Work out the finished part from the listing and answer in its coordinate system (mm). Face numbers are marked on the shaded views. A direction names the side the tool comes from. Give positions to 0.01 mm unless a question says otherwise; leave off trailing zeros. Order: outer loops, then holes, each group sorted by start corner. A loop starts at its lowest first (then second) coordinate and runs counter-clockwise, first axis right, second up. Notation, with made-up numbers: M -18.5,14 L -14.5,14 A18 cw -14.5,40 Z; hole C 44.5,-11.75 d3. An arc over 180 degrees is marked long. One line per item, written item: value.
from build123d import *

# Parameters (mm, degrees)
SKETCH1_W             = 76.2
SKETCH1_H             = 203.2
BOSS_EXTRUDE1_DEPTH   = 6.35
BOSS_EXTRUDE1_2_DEPTH = 6.35
SKETCH2_W             = 38.1
SKETCH2_H             = 76.2
BOSS_EXTRUDE2_DEPTH   = 889
SKETCH3_W             = 177.8
SKETCH3_H             = 38.1
BOSS_EXTRUDE3_DEPTH   = 76.2
SKETCH4_R             = 4.2
CUT_EXTRUDE1_DEPTH    = 180
SKETCH5_R             = 2.6
CUT_EXTRUDE2_DEPTH    = 10
SKETCH6_W             = 25
SKETCH6_H             = 18
BOSS_EXTRUDE4_DEPTH   = 10
SKETCH7_W             = 177.8
SKETCH7_H             = 19
BOSS_EXTRUDE5_DEPTH   = 2.54


with BuildPart() as part:
    # Sketch1 → Boss-Extrude1 (new body)
    with BuildSketch(Plane(origin=(0, 0, 0), x_dir=(1, 0, 0), z_dir=(0, 1, 0))):
        with Locations((127, -101.6)):
            Rectangle(SKETCH1_W, SKETCH1_H)
    extrude(amount=BOSS_EXTRUDE1_DEPTH)



with BuildPart() as body_2:
    # Sketch1 → Boss-Extrude1 2 (new body)
    with BuildSketch(Plane(origin=(0, 0, 0), x_dir=(1, 0, 0), z_dir=(0, 1, 0))):
        with Locations((-127, -101.6)):
            Rectangle(SKETCH1_W, SKETCH1_H)
    extrude(amount=BOSS_EXTRUDE1_2_DEPTH)


with BuildPart() as part_1:
    add(part.part)

    add(body_2.part)  # Boss-Extrude2 merges body 2
    # Sketch2 → Boss-Extrude2 (add)
    with BuildSketch(Plane(origin=(0, 6.35, 0), x_dir=(1, 0, 0), z_dir=(0, 1, 0))):
        with Locations((-107.95, -101.6)):
            Rectangle(SKETCH2_W, SKETCH2_H)
        with Locations((107.95, -101.6)):
            Rectangle(SKETCH2_W, SKETCH2_H)
    extrude(amount=BOSS_EXTRUDE2_DEPTH)

    # Sketch3 → Boss-Extrude3 (add)
    with BuildSketch(Plane.XY.offset(139.7)):
        with Locations((0, 876.3)):
            Rectangle(SKETCH3_W, SKETCH3_H)
        with Locations((0, 711.2)):
            Rectangle(SKETCH3_W, SKETCH3_H)
    extrude(amount=-BOSS_EXTRUDE3_DEPTH)

    # Sketch4 → Cut-Extrude1 (cut)
    with BuildSketch(Plane(origin=(0, 895.35, 0), x_dir=(1, 0, 0), z_dir=(0, 1, 0))):
        with Locations(Location((0, -119.7, 0), (0, 0, 270))):
            Circle(SKETCH4_R)
    extrude(amount=-CUT_EXTRUDE1_DEPTH, mode=Mode.SUBTRACT)

    # Sketch5 → Cut-Extrude2 (cut)
    with BuildSketch(Plane.XZ.offset(-857.25)):
        with Locations(Location((-12, 119.7, 0), (0, 0, 270))):
            Circle(SKETCH5_R)
        with Locations(Location((12, 119.7, 0), (0, 0, 90))):
            Circle(SKETCH5_R)
    extrude(amount=-CUT_EXTRUDE2_DEPTH, mode=Mode.SUBTRACT)

    # Sketch6 → Boss-Extrude4 (add)
    with BuildSketch(Plane(origin=(0, 730.25, 0), x_dir=(1, 0, 0), z_dir=(0, 1, 0))):
        with Locations((52.5, -130.7)):
            Rectangle(SKETCH6_W, SKETCH6_H)
        with Locations((-52.5, -130.7)):
            Rectangle(SKETCH6_W, SKETCH6_H)
    extrude(amount=BOSS_EXTRUDE4_DEPTH)

    # Sketch7 → Boss-Extrude5 (add)
    with BuildSketch(Plane.XY.offset(139.7)):
        with Locations((0, 819.25)):
            Rectangle(SKETCH7_W, SKETCH7_H)
    extrude(amount=-BOSS_EXTRUDE5_DEPTH)


solid = part_1.part
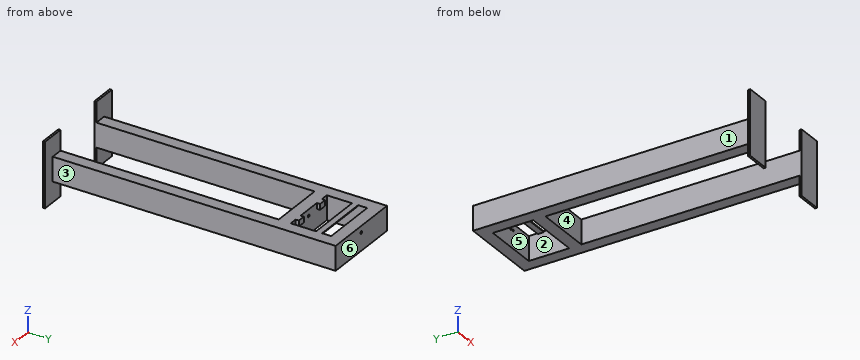
(1) Which of the six approach directions +Z, -Z, +X, -X, +Y, -Y give full straight-line access (tool end or side, diameter ignored) to the marked faces 4, 5 and 6?
Findings:
face 4: +Z, -Z, -Y
face 5: +Z, -Z
face 6: +Z, -Z, +X, -X, +Y
(2) Find the intervals of material crossed by probe 1 along X at (y, z) = (787, 65.5); probe 2 along X at (y, z) = (874, 119); probe 3 along X at (y, z) = (865, 119), in increasing order. Write a range as from..to.
Findings:
probe 1: x = -127..-88.9, 88.9..127
probe 2: x = -127..-4.14, 4.14..127
probe 3: x = -127..-14.5, -9.5..-4.14, 4.14..9.5, 14.5..127
(3) Section B-B, the plane z = 90 is taken. Give the vertices of the cut face in (x, y), then the cut area to 3 significant figures.
Findings:
outline: M -165.1,0 L -88.9,0 L -88.9,692.15 L 88.9,692.15 L 88.9,0 L 165.1,0 L 165.1,6.35 L 127,6.35 L 127,895.35 L -127,895.35 L -127,6.35 L -165.1,6.35 Z; hole M -88.9,730.25 L 88.9,730.25 L 88.9,857.25 L -88.9,857.25 Z
area: 82,300 mm^2
(4) Section C-C, the plane z = 173.5 is taken. Give the vertices of the cut face in (x, y), then the cut area to 3 significant figures.
Findings:
outline: M -165.1,0 L -88.9,0 L -88.9,6.35 L -165.1,6.35 Z; M 88.9,0 L 165.1,0 L 165.1,6.35 L 88.9,6.35 Z
area: 968 mm^2
(5) Section A-A, the plane y = 163.5 is taken. Give the vertices of the cut face in (x, z).
Findings:
outline: M -127,63.5 L -88.9,63.5 L -88.9,139.7 L -127,139.7 Z; M 88.9,63.5 L 127,63.5 L 127,139.7 L 88.9,139.7 Z
(6) Given P1, Ø0.8, axis at x = 41.5, z = 139, coming from the -Y side; P2, Ø1.5, axis at y = 337.5, z = 77, coming from the -X side; P3, Ø3, axis at y = 733.5, z = 130, coming from the +X side, each flat-ended and moving along its own axis, determine where each tip first touches the part or whether it passes through.
Findings:
P1: stops at y = 692.15
P2: stops at x = -127
P3: stops at x = 127
(7) Determine the mould class of the marked faces 1, 2 and 3 for opening direction X: pulls with the +X half, pulls with the -X half, needs draft (parallel to the pull), parting line crosses it, or undercut.
Findings:
face 1: pulls with the -X half
face 2: undercut
face 3: pulls with the +X half
